Autodesk Inventor part; units mm, degrees
ref_plane "YZ Plane" through (0, 0, 0) normal (1, 0, 0) x (0, 1, 0)
ref_plane "XZ Plane" through (0, 0, 0) normal (0, 1, 0) x (-1, 0, 0)
ref_plane "XY Plane" through (0, 0, 0) normal (0, 0, 1) x (1, 0, 0)
sketch "Schizzo3" plane through (0, 0, 0) normal (0, 0, 1) x (1, 0, 0)
  line L0 (-66.1458, 0) -> (66.1458, 0)
  line L1 (-4.2292, 27) -> (-4.2292, 13)
  line L2 (-4.2292, 13) -> (5.7708, 13)
  line L3 (5.7708, 13) -> (5.7708, 10)
  line L4 (-23.2292, 27) -> (-23.2292, 23.5)
  line L5 (-23.2292, 23.5) -> (-9.2292, 23.5)
  line L6 (-9.2292, 23.5) -> (-9.2292, 21)
  line L7 (-9.2292, 21) -> (-7.2292, 21)
  line L8 (-7.2292, 21) -> (-7.2292, 10)
  line L9 (-7.2292, 10) -> (5.7708, 10)
  line L10 (-23.2292, 27) -> (-4.2292, 27)
  point P0 (0, 0)
  point P1 (0, 0)
  dimension "d8" = 20
  dimension "d9" = 26
  dimension "d10" = 10
  dimension "d11" = 47
  dimension "d13" = 42
  dimension "d14" = 5
  dimension "d17" = 3
  dimension "d19" = 3.5
  dimension "d21" = 14
revolve "Rivoluzione1" add sketch "Schizzo3" angle 360 about axis through (-66.1458, 0, 0) along (1, 0, 0)
fillet "Raccordo1" radius 2 1 edges at (-4.2292, -13, 0)
chamfer "Smusso1" distance 0.5 angle 45 4 edges at (-23.2292, -23.5, 0) (-7.2292, -10, 0) (5.7708, -10, 0) (5.7708, -13, 0)
sketch "Schizzo4" plane through (-4.2292, 0, 0) normal (1, 0, 0) x (0, 0, -1)
  circle A0 centre (0, 0) radius 27
  circle A1 centre (0, 0) radius 27
  line L0 (-27, 0) -> (-27, 48)
  line L1 (-27, 48) -> (27, 48)
  line L2 (27, 48) -> (27, 0)
  dimension "d27" = 48
extrude "Estrusione3" add sketch "Schizzo4" against normal blind 9.5 contours A0 L0 L1 L2
chamfer "Smusso2" distance 0.5 angle 45 8 edges at (-4.2292, 24, 27) (-4.2292, -27, 0) (-4.2292, 24, -27) (-23.2292, -27, 0) (-4.2292, 48, 0) (-13.7292, 48, 0) (-8.9792, 48, -27) (-8.9792, 48, 27)
sketch "Schizzo5" plane through (-13.7292, 0, 0) normal (-1, 0, 0) x (0, 0, 1)
  line L0 (27, 0) -> (27, 47.5)
  line L1 (26.5, 48) -> (-26.5, 48)
  line L2 (-27, 47.5) -> (-27, 0)
  point P0 (0, 0)
  point P1 (13.5, 38)
  point P2 (-13.5, 38)
  dimension "d33" = 13.5
  dimension "d34" = 10
  dimension "d35" = 13.5
hole "Foro1" at (-13.7292, 38, 13.5) at (-13.7292, 38, -13.5) direction (1, 0, 0) diameter 10 end through all
properties part number "Porta cuscinetto puleggia operatrice" material "Acciaio inossidabile"
CAD build for the part. Positions are in the model's coordinates, mm. A direction names the side the tool comes from. Give positions to 0.01 mm unless a question says otherwise; leave off trailing zeros. Order: outer loops, then holes, each group sorted by start corner. A loop starts at its lowest first (then second) coordinate and runs counter-clockwise, first axis right, second up. Notation, with made-up numbers: (87.5, 69) - (99.5, 69) arc R16 ccw to (99.5, 84) - close; hole circle Ø6 at (-9, -22.5). An arc over 180 degrees is marked (long way). Write each question's results on one line, items separated by ' | '.
1. Saw through at A-A on y = 34. List the corners of the cut face in (x, z).
Calculated:
outline: (-13.73, -27) - (-4.73, -27) - (-4.23, -26.5) - (-4.23, -16.5) - (-13.73, -16.5) - close; (-13.73, -10.5) - (-4.23, -10.5) - (-4.23, 10.5) - (-13.73, 10.5) - close; (-13.73, 16.5) - (-4.23, 16.5) - (-4.23, 26.5) - (-4.73, 27) - (-13.73, 27) - close
2. Pin check, flat tips, straight feed: pin 1 (12 mm diameter, centred on y = 0, z = 0, fed in from +X); pin 2 (6 mm diameter, centred on x = -13, z = 16, fed in from -Y); pin 3 (2 mm diameter, centred on x = 2, y = 11, fed in from -Z); pin 4 (23.5 mm diameter, centred on y = -5.5, z = 1, fed in from -X). Stop position of each tip, or through.
Calculated:
pin 1: passes through | pin 2: stops at y = -23.66 | pin 3: stops at z = -8.31 | pin 4: stops at x = -7.23
3. Saw through at B-B on x = -11. List the corners of the cut face in (y, z).
Calculated:
outline: (0, -27) - (47.5, -27) - (48, -26.5) - (48, 26.5) - (47.5, 27) - (0, 27) arc R27 ccw to start; hole circle Ø47 at (0, 0); hole circle Ø10 at (38, -13.5); hole circle Ø10 at (38, 13.5)
4. Pull direction Y, two halves, no side cores. Call faces 4 (the face through (1.573, -10.316, -7.91)), 5 (the face through (-9, 24, -27)), 6 (the face through (-8.913, 33.784, 16.188)): released by +Y, released by -Y, zero draft, split by the parting line, or undercut.
Calculated:
face 4: split by the parting line | face 5: zero draft | face 6: undercut
5. 3-axis set-ups, long thin cutter, end or side, ignore diameter. For faces 1 (the face through (-4.229, 19, 0)), 2 (the face through (-4.372, -26.636, -0.586)), 3 (the face through (-9.229, -18, -12)): which of +Z, -Z, +X, -X, +Y, -Y reach the whole face in a straight line?
Calculated:
face 1: +X | face 2: +X, -Y | face 3: -X
6. Probe L1, parallel to Z at x = -7.75, y = 38; L2, parallel to Z at x = -8.75, y = 40; L3, parallel to Y at x = -8.25, z = 13.5. List the from-to ranges inside material, lowest first. Write a range as from..to.
Calculated:
L1: z = -27..-18.5, -8.5..8.5, 18.5..27 | L2: z = -27..-18.08, -8.92..8.92, 18.08..27 | L3: y = -23.38..-16.09, 16.09..33, 43..48
7. Saw through at C-C on x = -21.5. List the corners of the cut face in (y, z).
Calculated:
outline: circle Ø54 at (0, 0); hole circle Ø47 at (0, 0)
8. Saw through at D-D on x = -0.5. List the corners of the cut face in (y, z), and give its area (3 significant figures).
Calculated:
outline: circle Ø26 at (0, 0); hole circle Ø20 at (0, 0) | area: 217 mm2
